Input: part model. Units: mm. Frame: model coordinates. Face numbers are marked on the shaded views. A direction names the side the tool comes from. Round coordinates to 2 decimals unless told otherwise and drop trailing zeros. Write each loop counter-clockwise with the first axis right and the second up, starting at its lowest first coordinate (ties: lowest second). Pieces come first, ordered by that corner, then holes. Notation, with made-up numbers: (57, 8.5) -> (70, 8.5) arc R23 cw to (70, 34.5) -> close; hole circle Ø5 at (26.5, 26). An arc over 180 degrees is marked (long way). Write item = value, one per line.
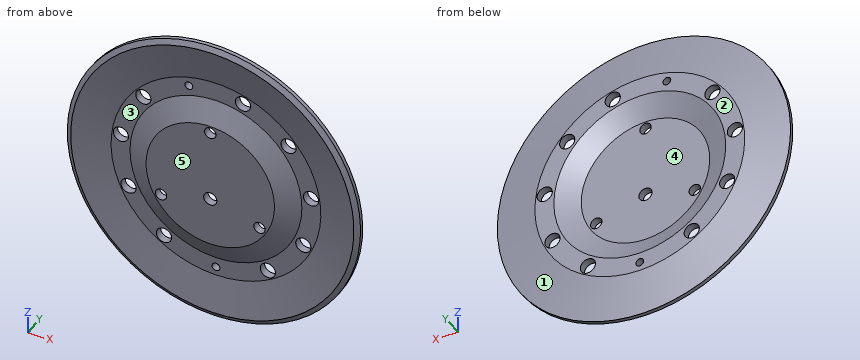
```python
from build123d import *

# Parameters (mm, degrees)
SKETCH_3_R          = 1.55
CUT_EXTRUDE_3_DEPTH = 83.322536404
SKETCH_4_R          = 3
CUT_EXTRUDE_5_DEPTH = 83.121860671
SKETCH_5_R          = 2.25
SKETCH_5_R_2        = 2.6
CUT_EXTRUDE_6_DEPTH = 83.322536404


with BuildPart() as part:
    # 草图1 → 旋转2 (revolve)
    with BuildSketch(Plane.XY, mode=Mode.PRIVATE) as revolve_2_sk:
        Polygon((25.421972318, 0), (34, 4), (41.5, 4), (56.009758155, 1.441538154), (58, 2.590604818), (58, 4.090604818), (41.5, 7), (34, 7), (25.421972318, 3), (0, 3), (0, 0), align=None)
    revolve(revolve_2_sk.sketch.rotate(Axis((0, 0, 0), (0, 1, 0)), 90), axis=Axis((0, 0, 0), (0, 1, 0)))

    # 草图3 → 切除-拉伸3 (cut, through all)
    with BuildSketch(Plane(origin=(0, 7, 0), x_dir=(1, 0, 0), z_dir=(0, 1, 0))):
        with Locations(Location((0, 38, 0), (0, 0, 270))):
            Circle(SKETCH_3_R)
        with Locations(Location((20.544351063, 31.967634248, 0), (0, 0, 270))):
            Circle(SKETCH_3_R)
        with Locations(Location((34.566015823, 15.785770494, 0), (0, 0, 270))):
            Circle(SKETCH_3_R)
        with Locations(Location((37.613214791, -5.407963854, 0), (0, 0, 270))):
            Circle(SKETCH_3_R)
        with Locations(Location((28.718483825, -24.88470789, 0), (0, 0, 270))):
            Circle(SKETCH_3_R)
        with Locations(Location((10.70583716, -36.460732997, 0), (0, 0, 270))):
            Circle(SKETCH_3_R)
        with Locations(Location((-10.70583716, -36.460732997, 0), (0, 0, 270))):
            Circle(SKETCH_3_R)
        with Locations(Location((-28.718483825, -24.88470789, 0), (0, 0, 270))):
            Circle(SKETCH_3_R)
        with Locations(Location((-37.613214791, -5.407963854, 0), (0, 0, 270))):
            Circle(SKETCH_3_R)
        with Locations(Location((-34.566015823, 15.785770494, 0), (0, 0, 270))):
            Circle(SKETCH_3_R)
        with Locations(Location((-20.544351063, 31.967634248, 0), (0, 0, 270))):
            Circle(SKETCH_3_R)
    extrude(amount=-CUT_EXTRUDE_3_DEPTH, mode=Mode.SUBTRACT)

    # 草图4 → 切除-拉伸5 (cut, through all)
    with BuildSketch(Plane.XZ.offset(-4)):
        with Locations((10.70583716, 36.460732997)):
            Circle(SKETCH_4_R)
        with Locations((28.718483825, 24.88470789)):
            Circle(SKETCH_4_R)
        with Locations((37.613214791, 5.407963854)):
            Circle(SKETCH_4_R)
        with Locations((-28.718483825, 24.88470789)):
            Circle(SKETCH_4_R)
        with Locations((-34.566015823, -15.785770494)):
            Circle(SKETCH_4_R)
        with Locations((-20.544351063, -31.967634248)):
            Circle(SKETCH_4_R)
        with Locations((20.544351063, -31.967634248)):
            Circle(SKETCH_4_R)
        with Locations((34.566015823, -15.785770494)):
            Circle(SKETCH_4_R)
        with Locations((-37.613214791, 5.407963854)):
            Circle(SKETCH_4_R)
    extrude(amount=-CUT_EXTRUDE_5_DEPTH, mode=Mode.SUBTRACT)

    # 草图5 → 切除-拉伸6 (cut, through all)
    with BuildSketch(Plane.XZ):
        with Locations((-19.485571585, -11.25)):
            Circle(SKETCH_5_R)
        with Locations((19.485571585, -11.25)):
            Circle(SKETCH_5_R)
        with Locations((0, 22.5)):
            Circle(SKETCH_5_R)
        with Locations((0, -5.95)):
            Circle(SKETCH_5_R_2)
    extrude(amount=-CUT_EXTRUDE_6_DEPTH, mode=Mode.SUBTRACT)


solid = part.part
```
1) Draft query along Z for the marked faces 1, 2 and 3. Return one class per face: +Z half, -Z half, draft (parallel to the pull), parting line (faces both ways), or undercut.
Solutions:
face_1 = parting line
face_2 = draft
face_3 = undercut
2) Cut plane B-B (z = 0). Return the cut outline in (x, y).
Solutions:
outline = (-58, 2.59) -> (-56.01, 1.44) -> (-41.5, 4) -> (-34, 4) -> (-25.42, 0) -> (25.42, 0) -> (34, 4) -> (41.5, 4) -> (56.01, 1.44) -> (58, 2.59) -> (58, 4.09) -> (41.5, 7) -> (34, 7) -> (25.42, 3) -> (-25.42, 3) -> (-34, 7) -> (-41.5, 7) -> (-58, 4.09) -> close
3) First-contact query: P1, Ø9.5, axis at x = 37.61, z = 5.41, coming from the -Y side; P2, Ø15.5, axis at x = 7, z = -0.5, coming from the +Y side; P3, Ø1, axis at x = -36, y = 1, coming from the +Z side. Flat tips, straight axial feed; report the tip coordinate or a pass-through.
Solutions:
P1 = 3.65
P2 = 3
P3 = 43.11
4) Cut plane A-A (x = 0). Count the separate pieces of the cut face and the enclosed holes in it, and give its area (3 significant figures).
Solutions:
separate_pieces = 4
enclosed_holes = 0
area = 307 mm^2
5) Line query: L1, parallel to Y at x = 39, z = 0.5; L2, parallel to Y at x = 12.5, z = 16.5; L3, parallel to Z at x = -51.5, y = 3.25. Output: solid intervals per line, ascending. Write a range as from..to.
Solutions:
L1 = 4..7
L2 = 0..3
L3 = -26.68..26.68
6) Access query for the marked faces 4 and 5. Directions: +Z, -Z, +X, -X, +Y, -Y. A direction counts if a zero-diameter tool reaches every point of the face in a straight line with its end or side. Return the directions, or none.
Solutions:
face_4 = +Y
face_5 = +Z, -Z, +X, -X, -Y
